CAD build for the part. Positions are in the model's coordinates, mm. A direction names the side the tool comes from. Coordinates: 2 decimals unless noted, no trailing zeros. Loops run counter-clockwise (first coordinate to the right, second up) from the corner with the lowest first, then second, coordinate; pieces in that order, holes last. Notation, with made-up numbers: (52, 52) -> (65, 52) arc R14 cw to (65, 68) -> close; hole circle Ø8 at (-10, 68.25). An arc over 180 degrees is marked (long way). Return JSON: item names as keys, results as strings. Group by question number.
(1) Tool access for faces 1 (the face through (2.96, 312.56, 229.64)), 2 (the face through (0, 210, 279)): list every direction of +Z, -Z, +X, -X, +Y, -Y with a clear straight run to the whole face (end or side of a thin tool).
(2) Mould opens along Z. For faces 3 (the face through (6, 210, 279)), 4 (the face through (2.958, 236.821, 227.646)), 5 (the face through (2.958, 276.146, 66.052)) say: pulls with the +Z half, pulls with the -Z half, needs draft (parallel to the pull), parting line crosses it, or undercut.
(3) Saw through at D-D on z = 183.5. Write the cut outline in (x, y).
(4) Saw through at C-C on y = 275. Write the cut outline in (x, z).
(5) Saw through at A-A on z = 315. Write the cut outline in (x, y), then the cut area to 3 significant figures.
(6) Saw through at B-B on x = 4.4. Write the cut outline in (y, z).
(7) Probe L1, parallel to Y at x = 2.3, z = 332; L2, parallel to Z at x = 1.55, y = 516.5; L3, parallel to Y at x = 2.45, z = 187. List the from-to ranges inside material, lowest first.
```python
from build123d import *

# Parameters (mm, degrees)
F1_DEPTH = 6


with BuildPart() as f1:
    # F0 (on Right) → F1 (new body)
    with BuildSketch(Plane.YZ):
        with BuildLine():
            Line((0, 574.042232), (0, -23.957768))
            Line((0, -23.957768), (550, -23.957768))
            Line((550, -23.957768), (550, 574.042232))
            Line((550, 574.042232), (295, 572.804987))
            Line((295, 572.804987), (295, 292.804987))
            Line((295, 292.804987), (330.622028, 164.675401))
            ThreePointArc((330.622028, 164.675401), (337.624821, 148.452911), (339.999926, 130.943851))
            ThreePointArc((339.999926, 130.943851), (274.713963, 66.042861), (210.001726, 131.515923))
            ThreePointArc((210.001726, 131.515923), (212.390971, 148.509617), (219.144239, 164.285786))
            Line((219.144239, 164.285786), (255, 292.804987))
            Line((255, 292.804987), (255, 572.804987))
            Line((255, 572.804987), (0, 574.042232))
        make_face()
    extrude(amount=F1_DEPTH)


solid = f1.part
```
Geometry results:
{
 "1": {"face 1": "+X, -X", "face 2": "+Z, -Z, -X, +Y, -Y"},
 "2": {"face 3": "needs draft", "face 4": "undercut", "face 5": "undercut"},
 "3": {"outline": "(0, 0) -> (6, 0) -> (6, 224.5) -> (0, 224.5) -> close; (0, 325.39) -> (6, 325.39) -> (6, 550) -> (0, 550) -> close"},
 "4": {"outline": "(0, -23.96) -> (6, -23.96) -> (6, 66.04) -> (0, 66.04) -> close"},
 "5": {"outline": "(0, 0) -> (6, 0) -> (6, 255) -> (0, 255) -> close; (0, 295) -> (6, 295) -> (6, 550) -> (0, 550) -> close", "area": "3,060 mm²"},
 "6": {"outline": "(0, -23.96) -> (550, -23.96) -> (550, 574.04) -> (295, 572.8) -> (295, 292.8) -> (330.62, 164.68) arc R65 cw to (340, 130.94) arc R65 cw (long way) to (210, 131.52) arc R65 cw to (219.14, 164.29) -> (255, 292.8) -> (255, 572.8) -> (0, 574.04) -> close"},
 "7": {"L1": "0 to 255, 295 to 550", "L2": "-23.96 to 573.88", "L3": "0 to 225.48, 324.42 to 550"}
}
